Geometry check sheet. Reference: drawing and pictorial views, mm from the part's lowest x, y, z. A direction names the side the tool comes from. Give positions to 0.01 mm unless a question says otherwise; leave off trailing zeros. Loops run counter-clockwise (first coordinate to the right, second up) from the corner with the lowest first, then second, coordinate; pieces in that order, holes last. Notation, with made-up numbers: M 23.5,33 L 79.5,33 A29 ccw 79.5,67 Z; hole C 8,5 d4. An arc over 180 degrees is marked long. One line per question, with ' | ' between items. Start each with the question number.
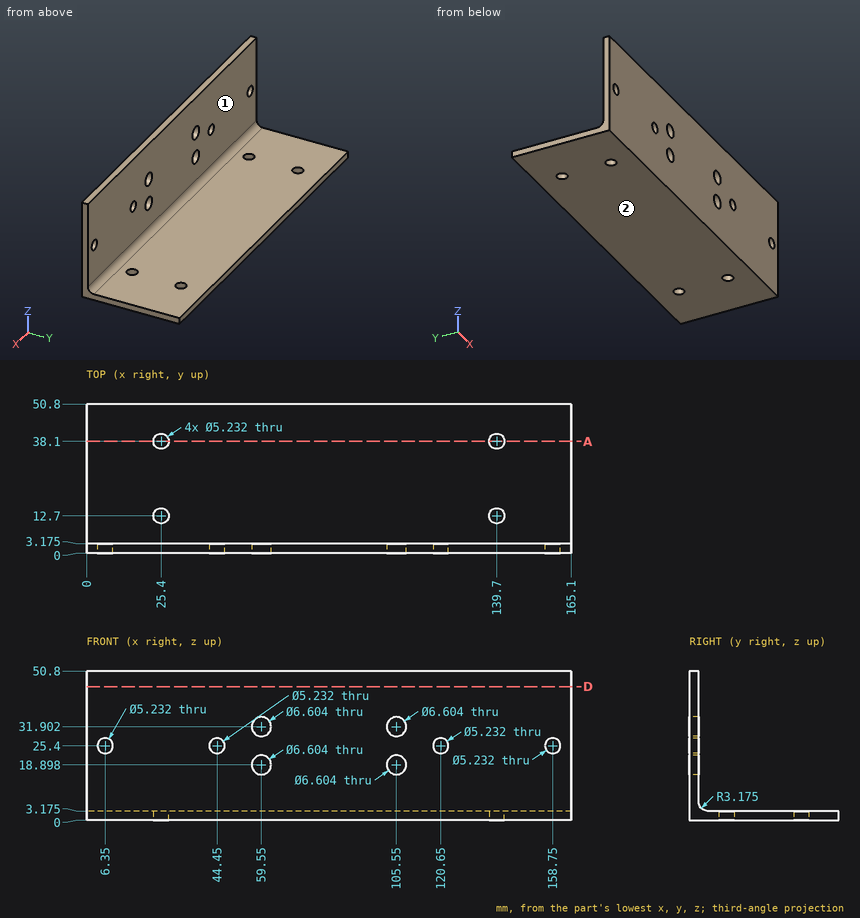
Q1. Cross-section at D-D (z = 45.5). Record the cut outline in (x, y) (1 decimal), and give its area (3 significant figures).
Q2. Access from +Z, -Z, +X, -X, +Y, -Y to the whole of each face (thin tool, end or side, straight path). Record for the marked faces 1 and 2.
Q3. Cross-section at A-A (y = 38.1). Record the cut outline in (x, z) (1 decimal), and give its area (3 significant figures).
Q4. Depth check by flat-ended pin: P1, Ø3, axis at x = 120.65, z = 25.4, coming from the -Y side; P2, Ø6, axis at x = 158.75, z = 25.4, coming from the +Y side (3 decimals); P3, Ø22, axis at x = 44, y = 37.5, coming from the +Z side (3 decimals). Enter the tip coordinate at first touch or a pass-through.
Q5. Material ranges on probe 1 along Y at (x, z) = (139.7, 1.7); probe 2 along X at (y, z) = (1, 25) (1 decimal); probe 3 along X at (y, z) = (1.95, 25.4), recorded low to high. Write a range as from..to.
Solved:
1) outline: M 0,0 L 165.1,0 L 165.1,3.2 L 0,3.2 Z | area: 524 mm²
2) face 1: +Z, +X, -X, +Y | face 2: -Z, +X, -X, +Y, -Y
3) outline: M 0,0 L 22.8,0 L 22.8,3.2 L 0,3.2 Z; M 28,0 L 137.1,0 L 137.1,3.2 L 28,3.2 Z; M 142.3,0 L 165.1,0 L 165.1,3.2 L 142.3,3.2 Z | area: 491 mm²
4) P1: passes through | P2: stops at y = 3.175 | P3: stops at z = 3.175
5) probe 1: y = 0..10.08, 15.32..35.48, 40.72..50.8 | probe 2: x = 0..3.8, 8.9..41.9, 47..118.1, 123.2..156.2, 161.3..165.1 | probe 3: x = 0..3.73, 8.97..41.83, 47.07..118.03, 123.27..156.13, 161.37..165.1
